from build123d import *

# Parameters (mm, degrees)
SKETCH1_W           = 55
SKETCH1_H           = 75
SKETCH1_R           = 1.32
BOSS_EXTRUDE1_DEPTH = 6
SKETCH2_R           = 3.25
CUT_EXTRUDE1_DEPTH  = 4


with BuildPart() as part:
    # Sketch1 → Boss-Extrude1 (new body)
    with BuildSketch(Plane.XY):
        with Locations((-27.5, -37.5)):
            Rectangle(SKETCH1_W, SKETCH1_H)
        with Locations((-43.375, -21.625)):
            Circle(SKETCH1_R, mode=Mode.SUBTRACT)
        with Locations((-11.625, -21.625)):
            Circle(SKETCH1_R, mode=Mode.SUBTRACT)
        with Locations((-11.625, -53.375)):
            Circle(SKETCH1_R, mode=Mode.SUBTRACT)
        with Locations((-43.375, -53.375)):
            Circle(SKETCH1_R, mode=Mode.SUBTRACT)
        with Locations((-27.5, -27.97)):
            Circle(SKETCH1_R, mode=Mode.SUBTRACT)
        with Locations((-27.5, -37.5)):
            Circle(SKETCH1_R, mode=Mode.SUBTRACT)
        with Locations((-27.5, -47.03)):
            Circle(SKETCH1_R, mode=Mode.SUBTRACT)
    extrude(amount=BOSS_EXTRUDE1_DEPTH)

    # Sketch2 → Cut-Extrude1 (cut)
    with BuildSketch(Plane(origin=(0, 0, 0), x_dir=(-1, 0, 0), z_dir=(0, 0, -1))):
        with Locations((11.625, -21.625)):
            Circle(SKETCH2_R)
        with Locations((43.375, -21.625)):
            Circle(SKETCH2_R)
        with Locations((43.375, -53.375)):
            Circle(SKETCH2_R)
        with Locations((11.625, -53.375)):
            Circle(SKETCH2_R)
    extrude(amount=-CUT_EXTRUDE1_DEPTH, mode=Mode.SUBTRACT)


solid = part.part
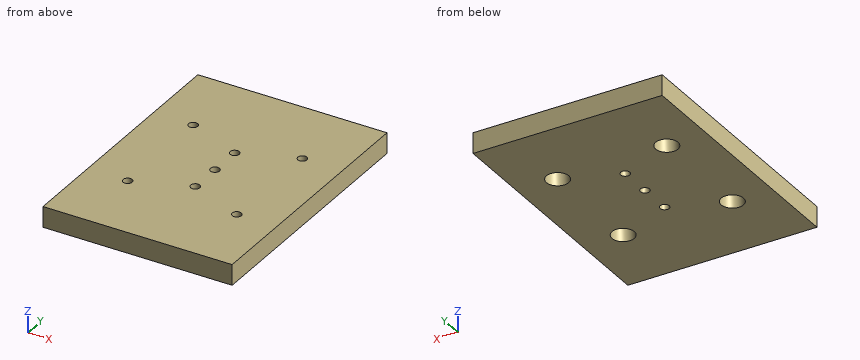
The listing builds one solid part. Answer for the finished solid, in the listing's coordinates (mm). Give positions to 0.01 mm unless a question says otherwise; leave off trailing zeros. Write each loop counter-clockwise with the first axis right and the second up, starting at its lowest first coordinate (ties: lowest second). Pieces come first, ordered by that corner, then holes.
Item 1: Find the intervals of material crossed by line 1 along Y through (x, z) = (-27.5, 1.45); line 2 along Y through (x, z) = (-45, 1.65); line 3 along X through (y, z) = (-21, 5.6), in increasing order.
Item 2: Section B-B, the plane x = -27.5 is taken. Write down the section's boundary in (y, z), plus the area to 3 significant figures.
Item 3: Section A-A, the plane y = -37.5 is taken. Write down the section's boundary in (x, z).
Item 4: Flat-ended cylindrical pins translate along their axes: P1, Ø3.5, axis at x = -27.5, y = -37.5, coming from the -Z side; P2, Ø3.5, axis at x = -43.375, y = -21.625, coming from the -Z side; P3, Ø2.5, axis at x = -11.625, y = -21.625, coming from the -Z side. Find the tip coordinate at first contact, or state that the pin passes through.
Item 5: Section C-C, the plane x = -43 is taken. Write down the section's boundary in (y, z).
Item 6: Section D-D, the plane z = 2.5 is taken. Write down the section's boundary in (x, y) (3 decimals).
Completed:
1. line 1: y = -75 to -48.35, -45.71 to -38.82, -36.18 to -29.29, -26.65 to 0
1. line 2: y = -75 to -56.19, -50.56 to -24.44, -18.81 to 0
1. line 3: x = -55 to -44.54, -42.21 to -12.79, -10.46 to 0
2. outline: (-75, 0) - (-48.35, 0) - (-48.35, 6) - (-75, 6) - close; (-45.71, 0) - (-38.82, 0) - (-38.82, 6) - (-45.71, 6) - close; (-36.18, 0) - (-29.29, 0) - (-29.29, 6) - (-36.18, 6) - close; (-26.65, 0) - (0, 0) - (0, 6) - (-26.65, 6) - close
2. area: 402 mm2
3. outline: (-55, 0) - (-28.82, 0) - (-28.82, 6) - (-55, 6) - close; (-26.18, 0) - (0, 0) - (0, 6) - (-26.18, 6) - close
4. P1: stops at z = 0
4. P2: stops at z = 4
4. P3: passes through
5. outline: (-75, 0) - (-56.6, 0) - (-56.6, 4) - (-54.64, 4) - (-54.64, 6) - (-75, 6) - close; (-52.11, 4) - (-50.15, 4) - (-50.15, 0) - (-24.85, 0) - (-24.85, 4) - (-22.89, 4) - (-22.89, 6) - (-52.11, 6) - close; (-20.36, 4) - (-18.4, 4) - (-18.4, 0) - (0, 0) - (0, 6) - (-20.36, 6) - close
6. outline: (-55, -75) - (0, -75) - (0, 0) - (-55, 0) - close; hole circle Ø6.5 at (-43.375, -53.375); hole circle Ø6.5 at (-43.375, -21.625); hole circle Ø2.64 at (-27.5, -47.03); hole circle Ø2.64 at (-27.5, -37.5); hole circle Ø2.64 at (-27.5, -27.97); hole circle Ø6.5 at (-11.625, -53.375); hole circle Ø6.5 at (-11.625, -21.625)
